For this review, take the finished solid that the model builds, in its own axes (mm). A direction names the side the tool comes from. Give positions to 0.01 mm unless a question says otherwise; leave off trailing zeros. Order: outer loops, then holes, each group sorted by start corner. A loop starts at its lowest first (then second) coordinate and runs counter-clockwise, first axis right, second up.
from build123d import *

# Parameters (mm, degrees)
BOSS_EXTRUDE1_DEPTH = 9
SKETCH3_R           = 1.5
CUT_EXTRUDE1_DEPTH  = 10
SKETCH8_W           = 5
SKETCH8_H           = 47
BOSS_EXTRUDE2_DEPTH = 38
SKETCH9_W           = 42
SKETCH9_H           = 5
BOSS_EXTRUDE3_DEPTH = 38
CUT_EXTRUDE2_DEPTH  = 38
SKETCH11_R          = 4
CUT_EXTRUDE3_DEPTH  = 5
CUT_EXTRUDE4_DEPTH  = 10
SKETCH13_R          = 1.5
CUT_EXTRUDE5_DEPTH  = 74.600271739
SKETCH14_R          = 3
CUT_EXTRUDE6_DEPTH  = 2
FILLET1_R           = 3


with BuildPart() as part:
    # Sketch2 → Boss-Extrude1 (new body)
    with BuildSketch(Plane.XY):
        with BuildLine():
            Line((0, 0), (0, 47))
            Line((0, 47), (47, 47))
            Line((47, 47), (47, 25.75))
            Line((47, 25.75), (31.68, 25.75))
            ThreePointArc((31.68, 25.75), (24.5283031, 28.175540714), (17, 27.58))
            Line((17, 27.58), (17, 0))
            Line((17, 0), (0, 0))
        make_face()
    extrude(amount=BOSS_EXTRUDE1_DEPTH)

    # Sketch3 → Cut-Extrude1 (cut)
    with BuildSketch(Plane.XY.offset(9)):
        with Locations((10.35, 5.65)):
            Circle(SKETCH3_R)
        with Locations((10.35, 36.65)):
            Circle(SKETCH3_R)
        with Locations((41.35, 36.65)):
            Circle(SKETCH3_R)
    extrude(amount=-CUT_EXTRUDE1_DEPTH, mode=Mode.SUBTRACT)

    # Sketch8 → Boss-Extrude2 (add)
    with BuildSketch(Plane(origin=(0, 0, 0), x_dir=(-1, 0, 0), z_dir=(0, 0, -1))):
        with Locations((-2.5, 23.5)):
            Rectangle(SKETCH8_W, SKETCH8_H)
    extrude(amount=BOSS_EXTRUDE2_DEPTH)

    # Sketch9 → Boss-Extrude3 (add)
    with BuildSketch(Plane(origin=(0, 0, 0), x_dir=(-1, 0, 0), z_dir=(0, 0, -1))):
        with Locations((-26, 44.5)):
            Rectangle(SKETCH9_W, SKETCH9_H)
    extrude(amount=BOSS_EXTRUDE3_DEPTH)

    # Sketch10 → Cut-Extrude2 (cut)
    with BuildSketch(Plane.ZY):
        Polygon((0, 0), (-23, 32), (-38, 32), (-38, 0), align=None)
    extrude(amount=-CUT_EXTRUDE2_DEPTH, mode=Mode.SUBTRACT)

    # Sketch11 → Cut-Extrude3 (cut)
    with BuildSketch(Plane.XY.offset(9)):
        with Locations((10, 20.85)):
            Circle(SKETCH11_R)
    extrude(amount=-CUT_EXTRUDE3_DEPTH, mode=Mode.SUBTRACT)

    # Sketch12 → Cut-Extrude4 (cut)
    with BuildSketch(Plane.XZ.offset(-42)):
        Polygon((47, -38), (47, -14), (27, -24.148784343), (27, -38), align=None)
    extrude(amount=-CUT_EXTRUDE4_DEPTH, mode=Mode.SUBTRACT)

    # Sketch13 → Cut-Extrude5 (cut, through all)
    with BuildSketch(Plane.XZ.offset(-42)):
        with Locations((37, -10)):
            Circle(SKETCH13_R)
    extrude(amount=-CUT_EXTRUDE5_DEPTH, mode=Mode.SUBTRACT)

    # Sketch14 → Cut-Extrude6 (cut)
    with BuildSketch(Plane(origin=(0, 42, 0), x_dir=(-1, 0, 0), z_dir=(0, -1, 0))):
        with Locations(Location((-37, 10, 0), (0, 0, 180))):
            Circle(SKETCH14_R)
    extrude(amount=-CUT_EXTRUDE6_DEPTH, mode=Mode.SUBTRACT)

    # Fillet1
    fillet1_edges = [part.edges().sort_by_distance(p)[0] for p in [
        (24.5283031, 28.175540714, 9),
        (0, 47, -14.5),
        (47, 47, -2.5),
        (47, 25.75, 4.5),
        (17, 27.58, 4.5),
        (17, 0, 4.5),
        (39.34, 25.75, 9),
        (47, 36.375, 9),
        (23.5, 47, 9),
        (0, 23.5, 9),
        (8.5, 0, 9),
        (17, 13.79, 9),
        (0, 16, -11.5),
        (0, 32, -30.5),
        (27, 47, -31.074392172),
        (37, 47, -19.074392172),
    ]]
    fillet(fillet1_edges, radius=FILLET1_R - 0.0001)  # a hair under: the kernel refuses the full size


solid = part.part
1) We need section A-A on y = 36.65. Give the boundary of the cut face in (x, z).
Answer sheet:
outline: (0, -38) - (5, -38) - (5, 0) - (8.85, 0) - (8.85, 9) - (3, 9) arc R3 ccw to (0, 6) - close; (11.85, 0) - (39.85, 0) - (39.85, 9) - (11.85, 9) - close; (42.85, 0) - (47, 0) - (47, 6) arc R3 ccw to (44, 9) - (42.85, 9) - close
2) Draft analysis for pull direction X (two halves, no side actions). For faces 5 (the face through (0.9, 46.14, -15.69)), 6 (the face through (46.14, 26.65, 3.04)), 7 (the face through (3.99, 15.78, -11.34)), 8 (the face through (40, 36, 5)), state which applies: +X half, -X half, draft (parallel to the pull), parting line (faces both ways), or undercut.
Answer sheet:
face 5: -X half
face 6: +X half
face 7: draft
face 8: undercut
3) We need section D-D on z = 3. Count the separate pieces of the cut face and the enclosed holes in it, then the cut area to 3 significant figures.
Answer sheet:
separate pieces: 1
enclosed holes: 3
area: 1,380 mm2
4) Clearance check with flat-ended pins moving along their axes: pin 1 (3 mm diameter, centred on x = 35.5, z = 2.5, fed in from -Y); pin 2 (5 mm diameter, centred on x = 10.35, y = 5.65, fed in from -Z); pin 3 (1.6 mm diameter, centred on y = 43, z = -32.5, fed in from +X); pin 4 (4 mm diameter, centred on x = 37, z = -10, fed in from +Y). State where each tip first meets the part, or that it passes through.
Answer sheet:
pin 1: stops at y = 25.75
pin 2: stops at z = 0
pin 3: stops at x = 27
pin 4: stops at y = 47
5) To check wall thickness, follow line 1 (X direction, y = 36, z = 4); line 2 (Y direction, x = 26, z = -3); line 3 (Y direction, x = 33.5, z = 0.5). State the ranges of each line that lie inside material, in increasing order.
Answer sheet:
line 1: x = 0 to 9, 11.7 to 40, 42.7 to 47
line 2: y = 42 to 47
line 3: y = 25.75 to 47
6) Tool access review of faces 1 (the face through (0.86, 32.9, -29.85)), 2 (the face through (9.133, 16.945, 6.535)), 3 (the face through (16.1, 13.93, 8.14)), 4 (the face through (4, 32, -30)): name each direction out of +Z, -Z, +X, -X, +Y, -Y from which nothing blocks a thin tool from reaching the whole face with its end or side.
Answer sheet:
face 1: -Z, -X, -Y
face 2: +Z
face 3: +Z, +X, -Y
face 4: -Z, +X, -X, -Y
7) We need section C-C on x = 10. Give the boundary of the cut face in (y, z), then the cut area to 3 significant figures.
Answer sheet:
outline: (0, 0) - (4.19, 0) - (4.19, 9) - (3, 9) arc R3 ccw to (0, 6) - close; (7.11, 0) - (35.19, 0) - (35.19, 9) - (24.85, 9) - (24.85, 4) - (16.85, 4) - (16.85, 9) - (7.11, 9) - close; (38.11, 0) - (42, 0) - (42, -38) - (47, -38) - (47, 6) arc R3 ccw to (44, 9) - (38.11, 9) - close
area: 517 mm2
8) We need section B-B on z = -26. Give the boundary of the cut face in (x, y).
Answer sheet:
outline: (0, 35) arc R3 ccw to (3, 32) - (5, 32) - (5, 42) - (27, 42) - (27, 44) arc R3 ccw to (24, 47) - (3, 47) arc R3 ccw to (0, 44) - close
